from build123d import *

# Parameters (mm, degrees)
SKETCH3_R               = 3.175
SKETCH3_R_2             = 3.429
BOSS_EXTRUDE1_DEPTH     = 77.47
CHAMFER1_SIZE           = 0.254
CUT_EXTRUDE1_DEPTH      = 145.117023717
CUT_EXTRUDE1_DEPTH_BACK = 145.117023717
SKETCH4_R               = 3.175
SKETCH4_R_2             = 3.429
SKETCH5_R               = 3.175
SKETCH5_R_2             = 12.7
CUT_EXTRUDE2_DEPTH      = 2.54
SKETCH6_R               = 3.175
CUT_EXTRUDE3_DEPTH      = 2.54


with BuildPart() as part:
    # Sketch3 → Boss-Extrude1 (new body)
    with BuildSketch(Plane.XY):
        with BuildLine():
            Line((107.95, -41.275), (-107.95, -41.275))
            ThreePointArc((-107.95, -41.275), (-112.440128061, -39.415128061), (-114.3, -34.925))
            Line((-114.3, -34.925), (-114.3, 34.925))
            ThreePointArc((-114.3, 34.925), (-112.440128061, 39.415128061), (-107.95, 41.275))
            Line((-107.95, 41.275), (107.95, 41.275))
            ThreePointArc((107.95, 41.275), (112.440128061, 39.415128061), (114.3, 34.925))
            Line((114.3, 34.925), (114.3, -34.925))
            ThreePointArc((114.3, -34.925), (112.440128061, -39.415128061), (107.95, -41.275))
        make_face()
        with Locations((-107.95, 34.925)):
            Circle(SKETCH3_R, mode=Mode.SUBTRACT)
        with Locations((-107.95, -34.925)):
            Circle(SKETCH3_R, mode=Mode.SUBTRACT)
        with Locations((107.95, -34.925)):
            Circle(SKETCH3_R, mode=Mode.SUBTRACT)
        with Locations((107.95, 34.925)):
            Circle(SKETCH3_R, mode=Mode.SUBTRACT)
        with Locations((-85.598, 0)):
            Circle(SKETCH3_R_2, mode=Mode.SUBTRACT)
        with Locations((85.598, 0)):
            Circle(SKETCH3_R_2, mode=Mode.SUBTRACT)
        with Locations((-15.875, 5.732638889)):
            Circle(SKETCH3_R, mode=Mode.SUBTRACT)
        with Locations((15.875, 5.732638889)):
            Circle(SKETCH3_R, mode=Mode.SUBTRACT)
        with Locations((15.875, -5.732638889)):
            Circle(SKETCH3_R, mode=Mode.SUBTRACT)
        with Locations((-15.875, -5.732638889)):
            Circle(SKETCH3_R, mode=Mode.SUBTRACT)
    extrude(amount=BOSS_EXTRUDE1_DEPTH)

    # Chamfer1
    chamfer1_edges = [part.edges().sort_by_distance(p)[0] for p in [
        (-112.440128061, 39.415128061, 77.47),
        (0, 41.275, 0),
        (112.440128061, 39.415128061, 0),
        (-114.3, 0, 77.47),
        (-112.440128061, -39.415128061, 77.47),
        (0, -41.275, 77.47),
        (112.440128061, -39.415128061, 77.47),
        (114.3, 0, 77.47),
        (112.440128061, 39.415128061, 77.47),
        (0, 41.275, 77.47),
        (114.3, 0, 0),
        (112.440128061, -39.415128061, 0),
        (0, -41.275, 0),
        (-112.440128061, -39.415128061, 0),
        (-114.3, 0, 0),
        (-112.440128061, 39.415128061, 0),
    ]]
    chamfer(chamfer1_edges, length=CHAMFER1_SIZE)

    # Sketch4 → Cut-Extrude1 (cut, two sides: drawn at the far end of the back side and taken through both)
    with BuildSketch(Plane.XY.offset(77.47).offset(-CUT_EXTRUDE1_DEPTH_BACK)):
        Polygon((111.76, 20.774487758), (93.799487758, 38.735), (-93.799487758, 38.735), (-111.76, 20.774487758), (-111.76, -20.774487758), (-93.799487758, -38.735), (93.799487758, -38.735), (111.76, -20.774487758), align=None)
        with Locations((-15.875, -5.732638889)):
            Circle(SKETCH4_R, mode=Mode.SUBTRACT)
        with Locations((15.875, -5.732638889)):
            Circle(SKETCH4_R, mode=Mode.SUBTRACT)
        with Locations((-85.598, 0)):
            Circle(SKETCH4_R_2, mode=Mode.SUBTRACT)
        with Locations((-15.875, 5.732638889)):
            Circle(SKETCH4_R, mode=Mode.SUBTRACT)
        with Locations((15.875, 5.732638889)):
            Circle(SKETCH4_R, mode=Mode.SUBTRACT)
        with Locations((85.598, 0)):
            Circle(SKETCH4_R_2, mode=Mode.SUBTRACT)
    extrude(amount=CUT_EXTRUDE1_DEPTH + CUT_EXTRUDE1_DEPTH_BACK, mode=Mode.SUBTRACT)

    # Sketch5 → Cut-Extrude2 (cut)
    with BuildSketch(Plane(origin=(0, 41.275, 0), x_dir=(1, 0, 0), z_dir=(0, 1, 0))):
        with Locations(Location((-88.483606557, -6.985, 0), (0, 0, 180))):
            Circle(SKETCH5_R)
        with Locations(Location((-63.083606557, -6.985, 0), (0, 0, 180))):
            Circle(SKETCH5_R)
        with Locations(Location((-63.083606557, -70.485, 0), (0, 0, 180))):
            Circle(SKETCH5_R)
        with Locations(Location((-88.483606557, -70.485, 0), (0, 0, 180))):
            Circle(SKETCH5_R)
        with Locations(Location((-75.783606557, -38.735, 0), (0, 0, 180))):
            Circle(SKETCH5_R_2)
    extrude(amount=-CUT_EXTRUDE2_DEPTH, mode=Mode.SUBTRACT)

    # Sketch6 → Cut-Extrude3 (cut)
    with BuildSketch(Plane(origin=(114.3, 0, 0), x_dir=(0, 0, -1), z_dir=(1, 0, 0))):
        with Locations((-57.785, 22.225)):
            Circle(SKETCH6_R)
        with Locations((-19.685, 22.225)):
            Circle(SKETCH6_R)
        with Locations((-19.685, -15.875)):
            Circle(SKETCH6_R)
        with Locations((-57.785, -15.875)):
            Circle(SKETCH6_R)
    extrude(amount=-CUT_EXTRUDE3_DEPTH, mode=Mode.SUBTRACT)


solid = part.part
Geometry check sheet. Reference: the model listing, model coordinates, mm. A direction names the side the tool comes from. Give positions to 0.01 mm unless a question says otherwise; leave off trailing zeros. Order: outer loops, then holes, each group sorted by start corner. A loop starts at its lowest first (then second) coordinate and runs counter-clockwise, first axis right, second up. Notation, with made-up numbers: M 43.25,66.5 L 85.25,66.5 A25 cw 85.25,88.5 Z; hole C 15.25,72 d3. An arc over 180 degrees is marked long. Use a Markdown table: item, result.
Item 1: Section check C-C (y = 3.5). Record the cut outline in (x, z).
Answers follow:
| item | result |
|---|---|
| outline | M -114.3,0.25 L -114.05,0 L -111.76,0 L -111.76,77.47 L -114.05,77.47 L -114.3,77.22 Z; M 111.76,0 L 114.05,0 L 114.3,0.25 L 114.3,77.22 L 114.05,77.47 L 111.76,77.47 Z |
Item 2: Draft check along Z on faces 6 (the cylindrical face through (113.048, -14.921, 16.657)), 7 (the conical face through (-112.3, -39.372, 77.345)), 8 (the flat face through (-2, 41.275, 38)). Enter one of: +Z half, -Z half, draft (parallel to the pull), parting line (faces both ways), or undercut.
Answers follow:
| item | result |
|---|---|
| face 6 | undercut |
| face 7 | +Z half |
| face 8 | draft |
Item 3: Section check D-D (z = 29.5). Record the cut outline in (x, y) (3 decimals).
Answers follow:
| item | result |
|---|---|
| outline | M -114.3,-34.925 A6.35 ccw -107.95,-41.275 L 107.95,-41.275 A6.35 ccw 114.3,-34.925 L 114.3,34.925 A6.35 ccw 107.95,41.275 L -67.066,41.275 L -67.066,38.735 L 93.799,38.735 L 111.76,20.774 L 111.76,-20.774 L 93.799,-38.735 L -93.799,-38.735 L -111.76,-20.774 L -111.76,20.774 L -93.799,38.735 L -84.502,38.735 L -84.502,41.275 L -107.95,41.275 A6.35 ccw -114.3,34.925 Z; hole C -107.95,-34.925 d6.35; hole C -107.95,34.925 d6.35; hole C 107.95,-34.925 d6.35; hole C 107.95,34.925 d6.35 |
Item 4: Section check B-B (z = 19). Record the cut outline in (x, y) (3 decimals).
Answers follow:
| item | result |
|---|---|
| outline | M -114.3,-34.925 A6.35 ccw -107.95,-41.275 L 107.95,-41.275 A6.35 ccw 114.3,-34.925 L 114.3,-18.975 L 111.76,-18.975 L 111.76,-20.774 L 93.799,-38.735 L -93.799,-38.735 L -111.76,-20.774 L -111.76,20.774 L -93.799,38.735 L 93.799,38.735 L 111.76,20.774 L 111.76,25.325 L 114.3,25.325 L 114.3,34.925 A6.35 ccw 107.95,41.275 L -107.95,41.275 A6.35 ccw -114.3,34.925 Z; M 111.76,-12.775 L 114.3,-12.775 L 114.3,19.125 L 111.76,19.125 Z; hole C -107.95,-34.925 d6.35; hole C -107.95,34.925 d6.35; hole C 107.95,-34.925 d6.35; hole C 107.95,34.925 d6.35 |
Item 5: Material ranges on line 1 along Y through (x, z) = (-80, 70) (3 decimals); line 2 along X through (y, z) = (8, 27.5); line 3 along Y through (x, z) = (107, 30) (3 decimals), recorded low to high.
Answers follow:
| item | result |
|---|---|
| line 1 | y = -41.275 to -38.735, 38.735 to 41.275 |
| line 2 | x = -114.3 to -111.76, 111.76 to 114.3 |
| line 3 | y = -41.275 to -37.955, -31.895 to -25.534, 25.534 to 31.895, 37.955 to 41.275 |
Item 6: Tool access check on faces 1 (the flat face through (111.76, 23, 20)), 2 (the cylindrical face through (-66.016, 40.023, 5.769)), 3 (the flat face through (102.654, -29.88, 38.193)), 4 (the conical face through (112.3, 39.372, 77.345)), 5 (the conical face through (-112.4, 39.28, 0.13)). Record the directions out of +Z, -Z, +X, -X, +Y, -Y that give a thin tool (end or side, any length) a straight path to the whole face; none if there is none.
Answers follow:
| item | result |
|---|---|
| face 1 | +X |
| face 2 | +Y |
| face 3 | +Z, -Z |
| face 4 | +Z, +X, +Y |
| face 5 | -Z, -X, +Y |
Item 7: Section check A-A (x = -44). Record the cut outline in (y, z) (3 decimals), and give its area (3 significant figures).
Answers follow:
| item | result |
|---|---|
| outline | M -41.275,0.254 L -41.021,0 L -38.735,0 L -38.735,77.47 L -41.021,77.47 L -41.275,77.216 Z; M 38.735,0 L 41.021,0 L 41.275,0.254 L 41.275,77.216 L 41.021,77.47 L 38.735,77.47 Z |
| area | 393 mm2 |
Item 8: Depth check by flat-ended pin: P1, Ø10, axis at x = -88.48, z = 6.98, coming from the +Y side (3 decimals); P2, Ø5.5, axis at x = -107.95, y = -34.925, coming from the -Z side; P3, Ø4, axis at y = 22.225, z = 19.685, coming from the +X side. Enter the tip coordinate at first touch or a pass-through.
Answers follow:
| item | result |
|---|---|
| P1 | stops at y = 41.275 |
| P2 | passes through |
| P3 | stops at x = 111.76 |
